Build history of the part. All positions in model axes, mm. A direction names the side the tool comes from. Round coordinates to 2 decimals unless told otherwise and drop trailing zeros. Loops run counter-clockwise (first coordinate to the right, second up) from the corner with the lowest first, then second, coordinate; pieces in that order, holes last. Notation, with made-up numbers: (72, -21.5) - (101, -21.5) arc R18 ccw to (101, -4.5) - close; hole circle Ø11 at (86, -19.75). An arc over 180 degrees is marked (long way). Use one line per item in the form item = value. Start each with the question number.
Q1. Drill centre lines: line 1 (X direction, y = -276.5, z = 321); line 2 (X direction, y = 99, z = -28); line 3 (X direction, y = 290.5, z = -316.5) (3 decimals). Where is each one in solid material? Low to high.
Q2. Pin check, flat tips, straight feed: pin 1 (4 mm diameter, centred on x = -435.5, y = -40, fed in from -Z); pin 2 (18 mm diameter, centred on x = 580, z = 118.5, fed in from -Y); pin 3 (3 mm diameter, centred on x = -62, z = 337.5, fed in from -Y). Stop position of each tip, or through.
Q3. Mould opens along Z. For faces 4 (the face through (564, -381, 148)), 5 (the face through (-773, -5, -368.3)), 6 (the face through (-772.124, -5.334, 353.814)), 7 (the face through (-4, -369, 339.725)) say: released by +Z, released by -Z, zero draft, split by the parting line, or undercut.
Q4. 3-axis set-ups, long thin cutter, end or side, ignore diameter. For faces 1 (the face through (-381, -2, 54)), 2 (the face through (773, -5, -368.3)), 3 (the face through (758.825, -30, -249)): which of +Z, -Z, +X, -X, +Y, -Y reach the whole face in a straight line?
Q5. Saw through at C-C (x = -175). Give the cut face in (y, z) (3 decimals).
Q6. Saw through at A-A (z = -277.5). Give the cut face in (x, y) (3 decimals).
Q7. Saw through at D-D (z = 204). Give the cut face in (x, y) (3 decimals).
Q8. Saw through at B-B (y = 21). Give the cut face in (x, z) (3 decimals), then the cut area to 3 significant figures.
```python
from build123d import *

# Parameters (mm, degrees)
F1_DEPTH = 381
F2_R     = 50.8
F3_W     = 660.4
F3_H     = 6.35
F4_DEPTH = 25.4
F3_W_2   = 371.475
F3_H_2   = 22.225
F5_DEPTH = 19.05
F6_R     = 6.35


with BuildPart() as f1:
    # F0 (on Front) → F1 (new body, symmetric)
    with BuildSketch(Plane.XZ):
        Polygon((787.4, 368.3), (-787.4, 368.3), (-787.4, -368.3), (-758.825, -368.3), (-758.825, -224.1076678038), (-381, -224.1076678038), (-381, 339.725), (-330.2, 339.725), (-330.2, 288.925), (330.2, 288.925), (330.2, 339.725), (381, 339.725), (381, -224.1076678038), (758.825, -224.1076678038), (758.825, -368.3), (787.4, -368.3), align=None)
    extrude(amount=F1_DEPTH, both=True)

    # F2
    f2_edges = [f1.edges().sort_by_distance(p)[0] for p in [
        (787.4, 0, 368.3),
        (-787.4, 0, 368.3),
    ]]
    fillet(f2_edges, radius=F2_R)

    # F3 (on face) → F4 (cut)
    with BuildSketch(Plane.XZ.offset(381)):
        Polygon((-758.825, 339.725), (-758.825, -224.1076678038), (-752.475, -224.1076678038), (-752.475, 104.775), (-752.475, 127), (-752.475, 168.275), (-381, 168.275), (-381, 174.625), (-752.475, 174.625), (-752.475, 269.875), (-752.475, 292.1), (-752.475, 333.375), (-381, 333.375), (-381, 339.725), align=None)
        with Locations((0, 336.55)):
            Rectangle(F3_W, F3_H)
        Polygon((758.825, 339.725), (381, 339.725), (381, 333.375), (752.475, 333.375), (752.475, 292.1), (752.475, 269.875), (752.475, 174.625), (381, 174.625), (381, 168.275), (752.475, 168.275), (752.475, 127), (752.475, 104.775), (752.475, -224.1076678038), (758.825, -224.1076678038), align=None)
    extrude(amount=-F4_DEPTH, mode=Mode.SUBTRACT)

    # F3 (on face) → F5 (cut)
    with BuildSketch(Plane.XZ.offset(381)):
        with Locations((-566.7375, 115.8875)):
            Rectangle(F3_W_2, F3_H_2)
        with Locations((-566.7375, 280.9875)):
            Rectangle(F3_W_2, F3_H_2)
        with Locations((566.7375, 280.9875)):
            Rectangle(F3_W_2, F3_H_2)
        with Locations((566.7375, 115.8875)):
            Rectangle(F3_W_2, F3_H_2)
    extrude(amount=-F5_DEPTH, mode=Mode.SUBTRACT)

    # F6
    f6_edges = [f1.edges().sort_by_distance(p)[0] for p in [
        (-566.7375, -381, -224.107668),
        (-381, -381, -59.666334),
        (-381, -381, 147.6375),
        (-381, -381, 222.25),
        (-566.7375, -381, 168.275),
        (-566.7375, -381, 174.625),
        (-381, -381, 312.7375),
        (-566.7375, -381, 333.375),
        (-752.475, -381, 312.7375),
        (-752.475, -381, 222.25),
        (-752.475, -381, 147.6375),
        (-752.475, -381, -59.666334),
        (-330.2, -381, 311.15),
        (0, -381, 288.925),
        (0, -381, 333.375),
        (330.2, -381, 311.15),
        (566.7375, -381, 333.375),
        (381, -381, 312.7375),
        (566.7375, -381, 292.1),
        (752.475, -381, 312.7375),
        (381, -381, 222.25),
        (566.7375, -381, 174.625),
        (752.475, -381, 222.25),
        (566.7375, -381, 168.275),
        (381, -381, 147.6375),
        (566.7375, -381, 127),
        (752.475, -381, 147.6375),
        (381, -381, -59.666334),
        (752.475, -381, -59.666334),
        (566.7375, -381, -224.107668),
    ]]
    fillet(f6_edges, radius=F6_R)


solid = f1.part
```
Report:
q1.line_1 = -787.28 to -381, -330.2 to 330.2, 381 to 787.28
q1.line_2 = -787.4 to -381, 381 to 787.4
q1.line_3 = -787.4 to -758.825, 758.825 to 787.4
q2.pin_1 = -224.11
q2.pin_2 = -377.12
q2.pin_3 = -355.6
q3.face_4 = zero draft
q3.face_5 = released by -Z
q3.face_6 = released by +Z
q3.face_7 = undercut
q4.face_1 = -Z, +Y, -Y
q4.face_2 = -Z, +X, -X, +Y, -Y
q4.face_3 = -Z, -Y
q5.outline = (-381, 295.275) arc R6.35 ccw to (-374.65, 288.925) - (381, 288.925) - (381, 368.3) - (-381, 368.3) - (-381, 339.725) - (-355.6, 339.725) - (-355.6, 333.375) - (-374.65, 333.375) arc R6.35 ccw to (-381, 327.025) - close
q6.outline = (-787.4, -381) - (-758.825, -381) - (-758.825, 381) - (-787.4, 381) - close; (758.825, -381) - (787.4, -381) - (787.4, 381) - (758.825, 381) - close
q7.outline = (-787.4, -381) - (-758.825, -381) - (-758.825, -355.6) - (-752.475, -355.6) - (-752.475, -374.65) arc R6.35 ccw to (-746.125, -381) - (-387.35, -381) arc R6.35 ccw to (-381, -374.65) - (-381, 381) - (-787.4, 381) - close; (381, -374.65) arc R6.35 ccw to (387.35, -381) - (746.125, -381) arc R6.35 ccw to (752.475, -374.65) - (752.475, -355.6) - (758.825, -355.6) - (758.825, -381) - (787.4, -381) - (787.4, 381) - (381, 381) - close
q8.outline = (-787.4, -368.3) - (-758.825, -368.3) - (-758.825, -224.108) - (-381, -224.108) - (-381, 339.725) - (-330.2, 339.725) - (-330.2, 288.925) - (330.2, 288.925) - (330.2, 339.725) - (381, 339.725) - (381, -224.108) - (758.825, -224.108) - (758.825, -368.3) - (787.4, -368.3) - (787.4, 317.5) arc R50.8 ccw to (736.6, 368.3) - (-736.6, 368.3) arc R50.8 ccw to (-787.4, 317.5) - close
q8.area = 544,000 mm²
